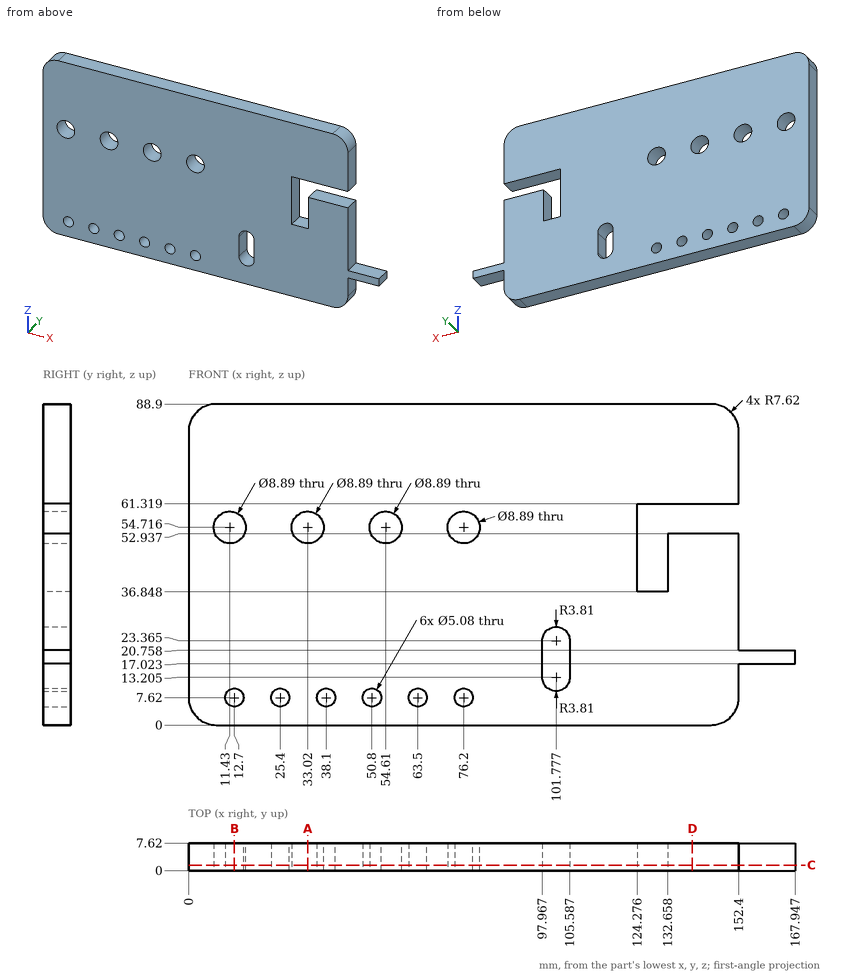
Job drawing, mm, ordinate dimensions from the low corner. One solid piece. Coordinates: 2 decimals unless noted, no trailing zeros. Loops run counter-clockwise (first coordinate to the right, second up) from the corner with the lowest first, then second, coordinate; pieces in that order, holes last. Notation, with made-up numbers: (-28.75, -39) - (11.25, -39) arc R19 ccw to (11.25, -24) - close; hole circle Ø9 at (46, 47). An arc over 180 degrees is marked (long way). Answer as a JSON object with one key per item and string values. Group by question number.
(1) Flat gauge pins, fed straight in: pin 1 (4.5 mm diameter, centred on x = 38.1, z = 7.62, fed in from -Y); pin 2 (4 mm diameter, centred on y = 4, z = 36, fed in from +X); pin 3 (4 mm diameter, centred on x = 158.5, y = 5.5, fed in from +Z). Where does each tip first touch, or does it go through?
(2) Cut at A-A (x = 33.02). Give the cut face in (y, z).
(3) Cut at C-C (y = 1.5). State how many separate pieces and enclosed holes the cut face has, then the cut area to 3 significant figures.
(4) Probe line 1 along Z through (x, y) = (63.5, 5.25); line 2 along Z through (x, y) = (12.7, 4) (1 decimal); line 3 along X through (y, z) = (6.25, 43.5). List the from-to ranges inside material, lowest first.
(5) Cut at D-D (x = 139.5). Give the cut face in (y, z).
(6) Cut at B-B (x = 12.7). Give the cut face in (y, z) (1 decimal).
Geometry says:
{
 "1": {"pin 1": "passes through", "pin 2": "stops at x = 152.4", "pin 3": "stops at z = 20.76"},
 "2": {"outline": "(0, 0) - (7.62, 0) - (7.62, 50.27) - (0, 50.27) - close; (0, 59.16) - (7.62, 59.16) - (7.62, 88.9) - (0, 88.9) - close"},
 "3": {"separate pieces": "1", "enclosed holes": "11", "area": "12,700 mm^2"},
 "4": {"line 1": "z = 0 to 5.08, 10.16 to 88.9", "line 2": "z = 0 to 5.1, 10.2 to 50.5, 59 to 88.9", "line 3": "x = 0 to 124.28, 132.66 to 152.4"},
 "5": {"outline": "(0, 0) - (7.62, 0) - (7.62, 52.94) - (0, 52.94) - close; (0, 61.32) - (7.62, 61.32) - (7.62, 88.9) - (0, 88.9) - close"},
 "6": {"outline": "(0, 0) - (7.6, 0) - (7.6, 5.1) - (0, 5.1) - close; (0, 10.2) - (7.6, 10.2) - (7.6, 50.5) - (0, 50.5) - close; (0, 59) - (7.6, 59) - (7.6, 88.9) - (0, 88.9) - close"}
}
